from build123d import *

# Parameters (mm, degrees)
EXTRUDE_THIN1_DEPTH = 238.125
FILLET1_R           = 0.889


with BuildPart() as part:
    # Sketch1 → Extrude-Thin1 (new body)
    with BuildSketch(Plane.XY):
        with BuildLine():
            Line((3.27025, 23.8125), (3.27025, 17.4625))
            Line((3.27025, 17.4625), (11.509375, 17.4625))
            Line((11.509375, 17.4625), (11.509375, 14.2875))
            Line((11.509375, 14.2875), (9.921875, 14.2875))
            Line((9.921875, 14.2875), (9.921875, 11.90625))
            ThreePointArc((9.921875, 11.90625), (6.489259214, 9.646453905), (5.159375, 5.757888938))
            Line((5.159375, 5.757888938), (5.159375, 3.175))
            Line((5.159375, 3.175), (3.571875, 3.175))
            Line((3.571875, 3.175), (3.571875, 0))
            Line((3.571875, 0), (-3.571875, 0))
            Line((-3.571875, 0), (-3.571875, 3.175))
            Line((-3.571875, 3.175), (-5.159375, 3.175))
            Line((-5.159375, 3.175), (-5.159375, 5.757888938))
            ThreePointArc((-5.159375, 5.757888938), (-6.489259214, 9.646453905), (-9.921875, 11.90625))
            Line((-9.921875, 11.90625), (-9.921875, 14.2875))
            Line((-9.921875, 14.2875), (-11.509375, 14.2875))
            Line((-11.509375, 14.2875), (-11.509375, 17.4625))
            Line((-11.509375, 17.4625), (-3.27025, 17.4625))
            Line((-3.27025, 17.4625), (-3.27025, 23.8125))
            Line((-3.27025, 23.8125), (-2.38125, 23.8125))
            Line((-2.38125, 23.8125), (-2.38125, 16.5735))
            Line((-2.38125, 16.5735), (-10.620375, 16.5735))
            Line((-10.620375, 16.5735), (-10.620375, 15.1765))
            Line((-10.620375, 15.1765), (-9.032875, 15.1765))
            Line((-9.032875, 15.1765), (-9.032875, 12.560099516))
            ThreePointArc((-9.032875, 12.560099516), (-5.579345299, 9.909740182), (-4.270375, 5.757888938))
            Line((-4.270375, 5.757888938), (-4.270375, 4.064))
            Line((-4.270375, 4.064), (-2.682875, 4.064))
            Line((-2.682875, 4.064), (-2.682875, 0.889))
            Line((-2.682875, 0.889), (2.682875, 0.889))
            Line((2.682875, 0.889), (2.682875, 4.064))
            Line((2.682875, 4.064), (4.270375, 4.064))
            Line((4.270375, 4.064), (4.270375, 5.757888938))
            ThreePointArc((4.270375, 5.757888938), (5.579345299, 9.909740182), (9.032875, 12.560099516))
            Line((9.032875, 12.560099516), (9.032875, 15.1765))
            Line((9.032875, 15.1765), (10.620375, 15.1765))
            Line((10.620375, 15.1765), (10.620375, 16.5735))
            Line((10.620375, 16.5735), (2.38125, 16.5735))
            Line((2.38125, 16.5735), (2.38125, 23.8125))
            Line((2.38125, 23.8125), (3.27025, 23.8125))
        make_face()
    extrude(amount=-EXTRUDE_THIN1_DEPTH)

    # Fillet1
    fillet1_edges = [part.edges().sort_by_distance(p)[0] for p in [
        (11.509375, 17.4625, -119.0625),
        (11.509375, 14.2875, -119.0625),
        (9.921875, 11.90625, -119.0625),
        (5.159375, 3.175, -119.0625),
        (3.571875, 0, -119.0625),
        (-3.571875, 0, -119.0625),
        (-5.159375, 3.175, -119.0625),
        (-9.921875, 11.90625, -119.0625),
        (-11.509375, 14.2875, -119.0625),
        (-11.509375, 17.4625, -119.0625),
        (-2.38125, 16.5735, -119.0625),
        (-9.032875, 15.1765, -119.0625),
        (-2.682875, 4.064, -119.0625),
        (2.682875, 4.064, -119.0625),
        (9.032875, 15.1765, -119.0625),
        (2.38125, 16.5735, -119.0625),
    ]]
    fillet(fillet1_edges, radius=FILLET1_R)


solid = part.part
Geometry check sheet. Reference: the model listing, model coordinates, mm. A direction names the side the tool comes from. Give positions to 0.01 mm unless a question says otherwise; leave off trailing zeros. Order: outer loops, then holes, each group sorted by start corner. A loop starts at its lowest first (then second) coordinate and runs counter-clockwise, first axis right, second up. Notation, with made-up numbers: M 86,-36 L 101,-36 A25 ccw 101,-22 Z; hole C 45,17 d6. An arc over 180 degrees is marked long. Use a Markdown table: item, result.
Item 1: Section check A-A (y = 8). Record the cut outline in (x, z) (3 decimals), and give its area (3 significant figures).
Answers follow:
| item | result |
|---|---|
| outline | M -5.568,-238.125 L -4.626,-238.125 L -4.626,0 L -5.568,0 Z; M 4.626,-238.125 L 5.568,-238.125 L 5.568,0 L 4.626,0 Z |
| area | 449 mm2 |
Item 2: Tool access check on faces 1 (the flat face through (7, 16.574, -117)), 2 (the flat face through (3.27, 21, -117)), 3 (the flat face through (-7, 17.462, -117)). Record the directions out of +Z, -Z, +X, -X, +Y, -Y that give a thin tool (end or side, any length) a straight path to the whole face; none if there is none.
Answers follow:
| item | result |
|---|---|
| face 1 | +Z, -Z |
| face 2 | +Z, -Z, +X, +Y |
| face 3 | +Z, -Z, -X, +Y |
Item 3: Material ranges on line 1 along Y through (x, z) = (-3.75, -160) (1 decimal); line 2 along X through (y, z) = (20, -171.5); line 3 along X through (y, z) = (16, -200), recorded low to high.
Answers follow:
| item | result |
|---|---|
| line 1 | y = 3.2 to 4.1, 16.6 to 17.5 |
| line 2 | x = -3.27 to -2.38, 2.38 to 3.27 |
| line 3 | x = -11.51 to -10.62, 10.62 to 11.51 |
Item 4: Depth check by flat-ended pin: P1, Ø0.6, axis at x = -10.5, z = -131, coming from the +Y side; P2, Ø2, axis at y = 2.5, z = -157.5, coming from the -X side; P3, Ø0.8, axis at y = 5.5, z = -126, coming from the -X side; P4, Ø8, axis at x = -3.5, z = -143, coming from the +Y side. Enter the tip coordinate at first touch or a pass-through.
Answers follow:
| item | result |
|---|---|
| P1 | stops at y = 17.46 |
| P2 | stops at x = -4.96 |
| P3 | stops at x = -5.16 |
| P4 | stops at y = 23.81 |
Item 5: Draft check along Y on faces 4 (the flat face through (7, 17.462, -117)), 5 (the cylindrical face through (-5.615, 9.96, -117.396)), 6 (the cylindrical face through (6.339, 9.444, -117.396)). Enter one of: +Y half, -Y half, draft (parallel to the pull), parting line (faces both ways), or undercut.
Answers follow:
| item | result |
|---|---|
| face 4 | +Y half |
| face 5 | undercut |
| face 6 | -Y half |
